Check sheet for the modelled part. Datum: model origin and axes. Units: mm. A direction names the side the tool comes from. Round coordinates to 2 decimals unless told otherwise and drop trailing zeros. Write each loop counter-clockwise with the first axis right and the second up, starting at its lowest first coordinate (ties: lowest second). Pieces come first, ordered by that corner, then holes. Notation, with made-up numbers: M -4.75,-29.5 L 47.25,-29.5 A23 cw 47.25,-4.5 Z; hole C -37.5,32.5 d6. An arc over 180 degrees is marked long. One line per item, written item: value.
from build123d import *

# Parameters (mm, degrees)
SKETCH_W                = 99
SKETCH_H                = 31
PAD_DEPTH               = 4
PAD001_DEPTH            = 11
PAD002_DEPTH            = 4
PAD001_MIRRORED_2_DEPTH = 11
POLARPATTERN_COUNT      = 2
CHAMFER_SIZE            = 0.99
FILLET_R                = 3
HOLE_D                  = 3.1
HOLE_DEPTH              = 25
HOLE_CSINK_D            = 7
HOLE_CSINK_ANGLE        = 90


with BuildPart() as part:
    # Sketch → Pad (new body)
    with BuildSketch(Plane.XY):
        Rectangle(SKETCH_W, SKETCH_H)
    extrude(amount=PAD_DEPTH)

    # Sketch001 → Pad001 (join)
    with BuildSketch(Plane.XY):
        Polygon((-49.5, 15.5), (-44.5, 15.5), (-44.5, 19.5), (-53.5, 19.5), (-53.5, 10.5), (-49.5, 10.5), align=None)
    pad001 = extrude(amount=PAD001_DEPTH)

    # Sketch002 → Pad002 (join)
    with BuildSketch(Plane.XY):
        Polygon((-47.5, 15.5), (-47.5, 20.5), (-23.5, 20.5), (-23.5, 15.5), (-28.5, 15.5), (-28.5, 17.5), (-42.5, 17.5), (-42.5, 15.5), align=None)
    pad002 = extrude(amount=PAD002_DEPTH)

    # Sketch001 Mirrored 2 → Pad001 Mirrored 2 (add)
    with BuildSketch(Plane(origin=(0, 0, 0), x_dir=(-1, 0, 0), z_dir=(0, 0, -1))):
        Polygon((-49.5, 15.5), (-44.5, 15.5), (-44.5, 19.5), (-53.5, 19.5), (-53.5, 10.5), (-49.5, 10.5), align=None)
    pad001_mirrored_2 = extrude(amount=-PAD001_MIRRORED_2_DEPTH)

    # PolarPattern: Pad001, Pad001 Mirrored 2 ×2 about axis
    polarpattern_axis = Axis((0, 0, 0), (0, 0, 1))
    for i in range(1, POLARPATTERN_COUNT):
        add(pad001.rotate(polarpattern_axis, i * 360 / POLARPATTERN_COUNT))
        add(pad001_mirrored_2.rotate(polarpattern_axis, i * 360 / POLARPATTERN_COUNT))

    # Mirrored001: Pad002 across Sketch002 H_Axis
    add(pad002.mirror(Plane.ZX))

    # Chamfer
    chamfer_edges = [part.edges().sort_by_distance(p)[0] for p in [
        (-47.5, -19.5, 2),
        (-47.5, 19.5, 2),
    ]]
    chamfer(chamfer_edges, length=CHAMFER_SIZE)

    # Fillet
    fillet_edges = [part.edges().sort_by_distance(p)[0] for p in [
        (-49.5, -15.5, 7.5),
        (-49.5, 15.5, 7.5),
        (49.5, 15.5, 7.5),
        (49.5, -15.5, 7.5),
    ]]
    fillet(fillet_edges, radius=FILLET_R)

    # Hole
    with Locations(Plane.XY.offset(4)):
        with Locations((-25, 0), (35, 0)):
            CounterSinkHole(HOLE_D / 2, HOLE_CSINK_D / 2, depth=HOLE_DEPTH, counter_sink_angle=HOLE_CSINK_ANGLE)


solid = part.part
Q1. Sectioned sample at B-B on z = 6.25. Enter the section's corners in (x, y).
Completed:
outline: M -53.5,-19.5 L -44.5,-19.5 L -44.5,-15.5 L -46.5,-15.5 A3 cw -49.5,-12.5 L -49.5,-10.5 L -53.5,-10.5 Z; M -53.5,10.5 L -49.5,10.5 L -49.5,12.5 A3 cw -46.5,15.5 L -44.5,15.5 L -44.5,19.5 L -53.5,19.5 Z; M 44.5,-19.5 L 53.5,-19.5 L 53.5,-10.5 L 49.5,-10.5 L 49.5,-12.5 A3 cw 46.5,-15.5 L 44.5,-15.5 Z; M 44.5,15.5 L 46.5,15.5 A3 cw 49.5,12.5 L 49.5,10.5 L 53.5,10.5 L 53.5,19.5 L 44.5,19.5 Z
Q2. Scan lines: line 1 (X direction, y = 0, z = 0.55); line 2 (Y direction, x = 35, z = 0.6); line 3 (X direction, y = -17, z = 7.75). Record each from-to range of solid material in increasing order. Write a range as [from, to].
Completed:
line 1: [-49.5, -26.55], [-23.45, 33.45], [36.55, 49.5]
line 2: [-15.5, -1.55], [1.55, 15.5]
line 3: [-53.5, -44.5], [44.5, 53.5]
Q3. Draft check along X on faces 5 (the flat face through (-53.5, 15, 5)), 6 (the flat face through (53.5, 15, 5)), 7 (the flat face through (44.5, 17, 5)). Enter one of: pulls with the +X half, pulls with the -X half, needs draft (parallel to the pull), parting line crosses it, or undercut.
Completed:
face 5: pulls with the -X half
face 6: pulls with the +X half
face 7: undercut
Q4. Access from +Z, -Z, +X, -X, +Y, -Y to the whole of each face (thin tool, end or side, straight path). Record for faces 1 (the flat face through (-49, -19.5, 7)), 2 (the flat face through (52, 10.5, 5)), 3 (the flat face through (-46, 15.5, 7)), 4 (the flat face through (-35, 17.5, 2)).
Completed:
face 1: +Z, -X, -Y
face 2: +Z, -Z, +X
face 3: +Z
face 4: +Z, -Z
Q5. Sectioned sample at A-A on x = -25. Enter the section's corners in (y, z), and give its area (3 significant figures).
Completed:
outline: M -20.5,0 L -1.55,0 L -1.55,2.05 L -3.5,4 L -20.5,4 Z; M 1.55,0 L 20.5,0 L 20.5,4 L 3.5,4 L 1.55,2.05 Z
area: 148 mm^2
Q6. Sectioned sample at D-D on x = 35. Enter the section's corners in (y, z).
Completed:
outline: M -15.5,0 L -1.55,0 L -1.55,2.05 L -3.5,4 L -15.5,4 Z; M 1.55,0 L 15.5,0 L 15.5,4 L 3.5,4 L 1.55,2.05 Z
Q7. Depth check by flat-ended pin: P1, Ø1.5, axis at x = -34.5, y = -15, coming from the +Z side; P2, Ø5, axis at y = -3, z = 2, coming from the -X side; P3, Ø3, axis at x = 26.5, z = 1, coming from the +Y side. Enter the tip coordinate at first touch or a pass-through.
Completed:
P1: z = 4
P2: x = -49.5
P3: y = 15.5
Q8. Sectioned sample at C-C on y = 0. Enter the section's corners in (x, z).
Completed:
outline: M -49.5,0 L -26.55,0 L -26.55,2.05 L -28.5,4 L -49.5,4 Z; M -23.45,0 L 33.45,0 L 33.45,2.05 L 31.5,4 L -21.5,4 L -23.45,2.05 Z; M 36.55,0 L 49.5,0 L 49.5,4 L 38.5,4 L 36.55,2.05 Z
